```python
from build123d import *

# Parameters (mm, degrees)
SKETCH_1_R      = 1.5
EXTRUDE_1_DEPTH = 3


with BuildPart() as part:
    # 草圖1 → 填料-伸長1 (new body)
    with BuildSketch(Plane(origin=(0, 3, 0), x_dir=(1, 0, 0), z_dir=(0, 1, 0))):
        with BuildLine():
            Line((-60, 57), (-60, -57))
            ThreePointArc((-60, -57), (-59.121320344, -59.121320344), (-57, -60))
            Line((-57, -60), (57, -60))
            ThreePointArc((57, -60), (59.121320344, -59.121320344), (60, -57))
            Line((60, -57), (60, 57))
            ThreePointArc((60, 57), (59.121320344, 59.121320344), (57, 60))
            Line((57, 60), (-57, 60))
            ThreePointArc((-57, 60), (-59.121320344, 59.121320344), (-60, 57))
        make_face()
        with Locations((52.5, -52.5)):
            Circle(SKETCH_1_R, mode=Mode.SUBTRACT)
        with Locations((-52.5, 52.5)):
            Circle(SKETCH_1_R, mode=Mode.SUBTRACT)
        with Locations((52.5, 52.5)):
            Circle(SKETCH_1_R, mode=Mode.SUBTRACT)
        with Locations((-52.5, -52.5)):
            Circle(SKETCH_1_R, mode=Mode.SUBTRACT)
        with BuildLine():
            Line((43.628679656, -39.128679656), (6.621320344, -2.121320344))
            ThreePointArc((6.621320344, -2.121320344), (5.742640687, 0), (6.621320344, 2.121320344))
            Line((6.621320344, 2.121320344), (43.628679656, 39.128679656))
            ThreePointArc((43.628679656, 39.128679656), (46.898050297, 39.77899791), (48.75, 37.007359313))
            Line((48.75, 37.007359313), (48.75, -37.007359313))
            ThreePointArc((48.75, -37.007359313), (46.898050297, -39.77899791), (43.628679656, -39.128679656))
        make_face(mode=Mode.SUBTRACT)
        with BuildLine():
            Line((39.128679656, 43.628679656), (2.121320344, 6.621320344))
            ThreePointArc((2.121320344, 6.621320344), (0, 5.742640687), (-2.121320344, 6.621320344))
            Line((-2.121320344, 6.621320344), (-39.128679656, 43.628679656))
            ThreePointArc((-39.128679656, 43.628679656), (-39.77899791, 46.898050297), (-37.007359313, 48.75))
            Line((-37.007359313, 48.75), (37.007359313, 48.75))
            ThreePointArc((37.007359313, 48.75), (39.77899791, 46.898050297), (39.128679656, 43.628679656))
        make_face(mode=Mode.SUBTRACT)
        with BuildLine():
            Line((-39.128679656, -43.628679656), (-2.121320344, -6.621320344))
            ThreePointArc((-2.121320344, -6.621320344), (0, -5.742640687), (2.121320344, -6.621320344))
            Line((2.121320344, -6.621320344), (39.128679656, -43.628679656))
            ThreePointArc((39.128679656, -43.628679656), (39.77899791, -46.898050297), (37.007359313, -48.75))
            Line((37.007359313, -48.75), (-37.007359313, -48.75))
            ThreePointArc((-37.007359313, -48.75), (-39.77899791, -46.898050297), (-39.128679656, -43.628679656))
        make_face(mode=Mode.SUBTRACT)
        with BuildLine():
            Line((-48.75, -37.007359313), (-48.75, 37.007359313))
            ThreePointArc((-48.75, 37.007359313), (-46.898050297, 39.77899791), (-43.628679656, 39.128679656))
            Line((-43.628679656, 39.128679656), (-6.621320344, 2.121320344))
            ThreePointArc((-6.621320344, 2.121320344), (-5.742640687, 0), (-6.621320344, -2.121320344))
            Line((-6.621320344, -2.121320344), (-43.628679656, -39.128679656))
            ThreePointArc((-43.628679656, -39.128679656), (-46.898050297, -39.77899791), (-48.75, -37.007359313))
        make_face(mode=Mode.SUBTRACT)
    extrude(amount=-EXTRUDE_1_DEPTH)


solid = part.part
```
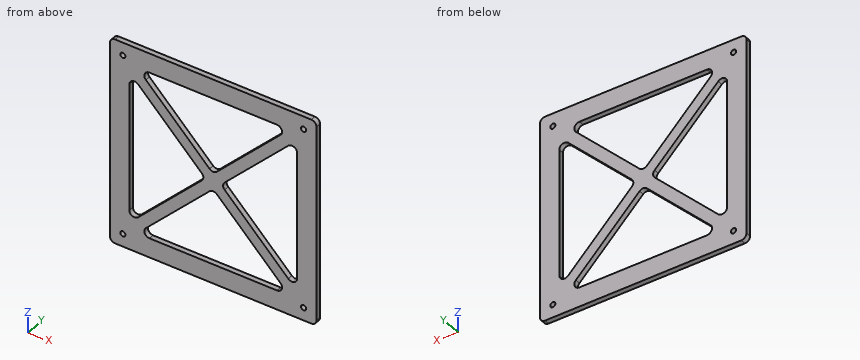
Part model, mm, in its own coordinate system. Round coordinates to 2 decimals unless told otherwise and drop trailing zeros. Loops run counter-clockwise (first coordinate to the right, second up) from the corner with the lowest first, then second, coordinate; pieces in that order, holes last.
1. Flat gauge pin, fed straight in: pin 1 (2.5 mm diameter, centred on x = -52.5, z = -52.5, fed in from +Y). Where does the tip first touch, or does it go through?
Solutions:
pin 1: passes through
2. Slice it at B-B (x = 23). Give the cut face in (y, z).
Solutions:
outline: (0, -60) - (3, -60) - (3, -48.75) - (0, -48.75) - close; (0, -27.5) - (3, -27.5) - (3, -18.5) - (0, -18.5) - close; (0, 18.5) - (3, 18.5) - (3, 27.5) - (0, 27.5) - close; (0, 48.75) - (3, 48.75) - (3, 60) - (0, 60) - close
3. Slice it at A-A (z = 10). Give the cut face in (x, y).
Solutions:
outline: (-60, 0) - (-48.75, 0) - (-48.75, 3) - (-60, 3) - close; (-14.5, 0) - (-5.5, 0) - (-5.5, 3) - (-14.5, 3) - close; (5.5, 0) - (14.5, 0) - (14.5, 3) - (5.5, 3) - close; (48.75, 0) - (60, 0) - (60, 3) - (48.75, 3) - close
4. Slice it at C-C (z = -52.5). Give the cut face in (x, y).
Solutions:
outline: (-60, 0) - (-54, 0) - (-54, 3) - (-60, 3) - close; (-51, 0) - (51, 0) - (51, 3) - (-51, 3) - close; (54, 0) - (60, 0) - (60, 3) - (54, 3) - close
5. Drill centre lines: line 1 along X through (y, z) = (1.7, 52.5); line 2 along X through (y, z) = (1.4, -11). Where is each one in solid material? Low to high.
Solutions:
line 1: x = -60 to -54, -51 to 51, 54 to 60
line 2: x = -60 to -48.75, -15.5 to -6.5, 6.5 to 15.5, 48.75 to 60
6. Slice it at D-D (x = -52.5). Give the cut face in (y, z).
Solutions:
outline: (0, -60) - (3, -60) - (3, -54) - (0, -54) - close; (0, -51) - (3, -51) - (3, 51) - (0, 51) - close; (0, 54) - (3, 54) - (3, 60) - (0, 60) - close
